Autodesk Inventor part; units mm, degrees
ref_plane "YZ Plane" through (0, 0, 0) normal (1, 0, 0) x (0, 1, 0)
ref_plane "XZ Plane" through (0, 0, 0) normal (0, 1, 0) x (-1, 0, 0)
ref_plane "XY Plane" through (0, 0, 0) normal (0, 0, 1) x (1, 0, 0)
sketch "Boceto1" plane through (0, 0, 0) normal (0, 1, 0) x (-1, 0, 0)
  circle A0 centre (0, 0) radius 75
  line L0 (65, -22) -> (41, -22)
  line L1 (41, -22) -> (41, 22)
  line L2 (41, 22) -> (65, 22)
  line L3 (65, 22) -> (65, -22)
  line L4 (37.6072, -39) -> (12.6072, -39)
  line L5 (12.6072, -39) -> (12.6072, -36)
  line L6 (12.6072, -36) -> (37.6072, -36)
  line L7 (37.6072, -36) -> (37.6072, -39)
  line L8 (37.6072, -45) -> (12.6072, -45)
  line L9 (12.6072, -45) -> (12.6072, -42)
  line L10 (12.6072, -42) -> (37.6072, -42)
  line L11 (37.6072, -42) -> (37.6072, -45)
  line L12 (35, -51) -> (10, -51)
  line L13 (10, -51) -> (10, -48)
  line L14 (10, -48) -> (35, -48)
  line L15 (35, -48) -> (35, -51)
  line L16 (35, -33) -> (10, -33)
  line L17 (10, -33) -> (10, -30)
  line L18 (10, -30) -> (35, -30)
  line L19 (35, -30) -> (35, -33)
  line L20 (-37.6072, -39) -> (-12.6072, -39)
  line L21 (-12.6072, -39) -> (-12.6072, -36)
  line L22 (-12.6072, -36) -> (-37.6072, -36)
  line L23 (-37.6072, -36) -> (-37.6072, -39)
  line L24 (-37.6072, -45) -> (-12.6072, -45)
  line L25 (-37.6072, -42) -> (-37.6072, -45)
  line L26 (-12.6072, -42) -> (-37.6072, -42)
  line L27 (-12.6072, -45) -> (-12.6072, -42)
  line L28 (-35, -51) -> (-10, -51)
  line L29 (-35, -48) -> (-35, -51)
  line L30 (-10, -48) -> (-35, -48)
  line L31 (-10, -51) -> (-10, -48)
  line L32 (-35, -33) -> (-10, -33)
  line L33 (-35, -30) -> (-35, -33)
  line L34 (-10, -30) -> (-35, -30)
  line L35 (-10, -33) -> (-10, -30)
  line L36 (-65, -22) -> (-41, -22)
  line L37 (-41, -22) -> (-41, 22)
  line L38 (-41, 22) -> (-65, 22)
  line L39 (-65, 22) -> (-65, -22)
  line L40 (37.6072, 39) -> (12.6072, 39)
  line L41 (12.6072, 39) -> (12.6072, 36)
  line L42 (12.6072, 36) -> (37.6072, 36)
  line L43 (37.6072, 36) -> (37.6072, 39)
  line L44 (37.6072, 45) -> (12.6072, 45)
  line L45 (37.6072, 42) -> (37.6072, 45)
  line L46 (12.6072, 42) -> (37.6072, 42)
  line L47 (12.6072, 45) -> (12.6072, 42)
  line L48 (35, 51) -> (10, 51)
  line L49 (35, 48) -> (35, 51)
  line L50 (10, 48) -> (35, 48)
  line L51 (10, 51) -> (10, 48)
  line L52 (35, 33) -> (10, 33)
  line L53 (35, 30) -> (35, 33)
  line L54 (10, 30) -> (35, 30)
  line L55 (10, 33) -> (10, 30)
  line L56 (-35, 30) -> (-35, 33)
  line L57 (-10, 33) -> (-10, 30)
  line L58 (-10, 30) -> (-35, 30)
  line L59 (-35, 33) -> (-10, 33)
  line L60 (-12.6072, 39) -> (-12.6072, 36)
  line L61 (-12.6072, 36) -> (-37.6072, 36)
  line L62 (-37.6072, 36) -> (-37.6072, 39)
  line L63 (-37.6072, 39) -> (-12.6072, 39)
  line L64 (-12.6072, 45) -> (-12.6072, 42)
  line L65 (-12.6072, 42) -> (-37.6072, 42)
  line L66 (-37.6072, 45) -> (-12.6072, 45)
  line L67 (-10, 48) -> (-35, 48)
  line L68 (-35, 51) -> (-10, 51)
  line L69 (-10, 51) -> (-10, 48)
  line L70 (-37.6072, 42) -> (-37.6072, 45)
  line L71 (-35, 48) -> (-35, 51)
  point P0 (0, 25.3749)
  dimension "d0" = 150
  dimension "d1" = 24
  dimension "d2" = 44
  dimension "d3" = 10
  dimension "d4" = 25
  dimension "d5" = 3
  dimension "d6" = 25
  dimension "d7" = 3
  dimension "d8" = 25
  dimension "d9" = 3
  dimension "d10" = 25
  dimension "d11" = 3
  dimension "d12" = 3
  dimension "d13" = 3
  dimension "d14" = 3
  dimension "d15" = 0
extrude "Extrusión1" add sketch "Boceto1" along normal blind 1.5
sketch "Boceto2" plane through (0, 1.5, 0) normal (0, 1, 0) x (1, 0, 0)
  line L0 (0, 0) -> (0, -9.9603)
  line L1 (0, 0) -> (61.7788, -62.8893)
  circle A0 centre (47.0174, -47.8626) radius 0.75
  arc A1 (50.5529, -44.327) -> (43.5135, -51.4295) centre (47.0174, -47.8626) ccw
  line L2 (-72.438, 0) -> (-75, 0)
  circle A2 centre (0, 0) radius 72.438
  line L3 (44.0781, -44.8705) -> (47.0174, -47.8626)
  line L4 (43.4505, -51.3665) -> (48.0344, -55.9504)
  line L5 (43.4505, -51.3665) -> (49.9332, -51.3665) construction
  line L6 (47.0174, -47.8626) -> (52.0174, -47.8626) construction
  line L7 (50.5529, -44.327) -> (55.1054, -48.8795)
  line L8 (55.1054, -48.8795) -> (48.0344, -55.9504)
  circle A3 centre (-47.0174, -47.8626) radius 0.75
  arc A4 (-43.5135, -51.4295) -> (-50.5529, -44.327) centre (-47.0174, -47.8626) ccw
  line L9 (-44.0781, -44.8705) -> (-47.0174, -47.8626)
  line L10 (-43.4505, -51.3665) -> (-48.0344, -55.9504)
  line L11 (-43.4505, -51.3665) -> (-49.9332, -51.3665) construction
  line L12 (-47.0174, -47.8626) -> (-52.0174, -47.8626) construction
  line L13 (-50.5529, -44.327) -> (-55.1054, -48.8795)
  line L14 (-55.1054, -48.8795) -> (-48.0344, -55.9504)
  line L15 (0, 0) -> (7.916, 0)
  line L16 (-44.0781, 44.8705) -> (-47.0174, 47.8626)
  circle A5 centre (-47.0174, 47.8626) radius 0.75
  line L17 (-43.4505, 51.3665) -> (-49.9332, 51.3665) construction
  arc A6 (-50.5529, 44.327) -> (-43.5135, 51.4295) centre (-47.0174, 47.8626) ccw
  line L18 (-43.4505, 51.3665) -> (-48.0344, 55.9504)
  line L19 (-47.0174, 47.8626) -> (-52.0174, 47.8626) construction
  line L20 (-50.5529, 44.327) -> (-55.1054, 48.8795)
  line L21 (-55.1054, 48.8795) -> (-48.0344, 55.9504)
  line L22 (0, 0) -> (61.7788, 62.8893)
  circle A7 centre (0, 0) radius 72.438
  circle A8 centre (47.0174, 47.8626) radius 0.75
  arc A9 (43.5135, 51.4295) -> (50.5529, 44.327) centre (47.0174, 47.8626) ccw
  line L23 (44.0781, 44.8705) -> (47.0174, 47.8626)
  line L24 (43.4505, 51.3665) -> (48.0344, 55.9504)
  line L25 (47.0174, 47.8626) -> (52.0174, 47.8626) construction
  line L26 (55.1054, 48.8795) -> (48.0344, 55.9504)
  line L27 (50.5529, 44.327) -> (55.1054, 48.8795)
  line L28 (43.4505, 51.3665) -> (49.9332, 51.3665) construction
  dimension "d26" = 1.5
  dimension "d27" = 45
  dimension "d28" = 44.49
  dimension "d29" = 45.51
extrude "Extrusión2" cut sketch "Boceto2" against normal blind 10 contours A0 L1 | L1 A0 | A8 L22 | L22 A8 | A3 | A5
sketch "Boceto3" plane through (0, 0, 0) normal (0, -1, 0) x (1, 0, 0)
  line L0 (0, 0) -> (0, 96.9999)
  line L1 (0, 0) -> (57.8177, 0)
  circle A0 centre (6.75, 65) radius 1.25
  circle A1 centre (-6.75, 65) radius 1.25
  circle A2 centre (6.75, -65) radius 1.25
  circle A3 centre (-6.75, -65) radius 1.25
  dimension "d32" = 2.5
  dimension "d33" = 6.75
  dimension "d34" = 65
extrude "Extrusión3" cut sketch "Boceto3" against normal blind 10
sketch "Boceto4" plane through (0, 0, 0) normal (0, -1, 0) x (1, 0, 0)
  circle A0 centre (-36, 14) radius 1.25
  line L0 (0, 0) -> (0, 13.2611)
  line L1 (0, 0) -> (12.4525, 0)
  circle A1 centre (36, 14) radius 1.25
  circle A2 centre (-36, -14) radius 1.25
  circle A3 centre (36, -14) radius 1.25
  line L2 (-41, 22) -> (-41, -22)
  point P0 (0, -13.2611)
  dimension "d37" = 2.5
  dimension "d38" = 14
  dimension "d39" = 5
extrude "Extrusión4" cut sketch "Boceto4" against normal blind 10
properties part number "Base"
For this review, take the finished solid that the model builds, in its own axes (mm). Coordinates: 2 decimals unless noted, no trailing zeros. Order: outer loops, then holes, each group sorted by start corner. A loop starts at its lowest first (then second) coordinate and runs counter-clockwise, first axis right, second up. Notation, with made-up numbers: (60.5, 1) - (67.5, 1) arc R21 ccw to (67.5, 9) - close; hole circle Ø6 at (47.5, 14.5). An arc over 180 degrees is marked (long way). Answer as CSV lines item,"result". Start each with the question number.
1) Add section C-C (x = -62.5). State the section outline as (y, z) points.
2) Insertion check: P1, Ø0.8, axis at x = -18, y = 1, coming from the +Z side; P2, Ø0.8, axis at x = 23.5, y = 0.5, coming from the +Z side; P3, Ø2, axis at x = -36, z = 14, coming from the -Y side; P4, Ø0.8, axis at y = 0.5, z = -43, coming from the -X side. Each pin has a flat end and moves straight along its axis. Give the tip position at first contact, or say it passes through.
3) Add section B-B (x = 54.5). State the section outline as (y, z) points, then the cut area to 3 significant figures.
4) Add section A-A (z = 0). State the section outline as (x, y) points, then the cut area to 3 significant figures.
5) Add section D-D (z = 18). State the section outline as (x, y) points, then the cut area to 3 significant figures.
6) To check wall thickness, follow line 1 along X through (y, z) = (0.65, 1.5) (3 decimals); line 2 along Z through (x, y) = (6.75, 1.1); line 3 along Z through (x, y) = (47.5, 1.05). State the ranges of each line that lie inside material, in increasing order. Write a range as [from, to].
Result:
1,outline,"(0, -41.46) - (1.5, -41.46) - (1.5, -22) - (0, -22) - close; (0, 22) - (1.5, 22) - (1.5, 41.46) - (0, 41.46) - close"
2,P1,"z = 72.91"
2,P2,"z = 71.35"
2,P3,"through"
2,P4,"x = -61.73"
3,outline,"(0, -51.52) - (1.5, -51.52) - (1.5, -22) - (0, -22) - close; (0, 22) - (1.5, 22) - (1.5, 51.52) - (0, 51.52) - close"
3,area,"88.6 mm^2"
4,outline,"(-75, 0) - (-65, 0) - (-65, 1.5) - (-75, 1.5) - close; (-41, 0) - (41, 0) - (41, 1.5) - (-41, 1.5) - close; (65, 0) - (75, 0) - (75, 1.5) - (65, 1.5) - close"
4,area,"153 mm^2"
5,outline,"(-72.81, 0) - (-65, 0) - (-65, 1.5) - (-72.81, 1.5) - close; (-41, 0) - (41, 0) - (41, 1.5) - (-41, 1.5) - close; (65, 0) - (72.81, 0) - (72.81, 1.5) - (65, 1.5) - close"
5,area,"146 mm^2"
6,line 1,"[-74.985, -65], [-41, 41], [65, 74.985]"
6,line 2,"[-74.7, -66.25], [-63.75, 63.75], [66.25, 74.7]"
6,line 3,"[-58.04, -48.44], [-47.29, -22], [22, 47.29], [48.44, 58.04]"
